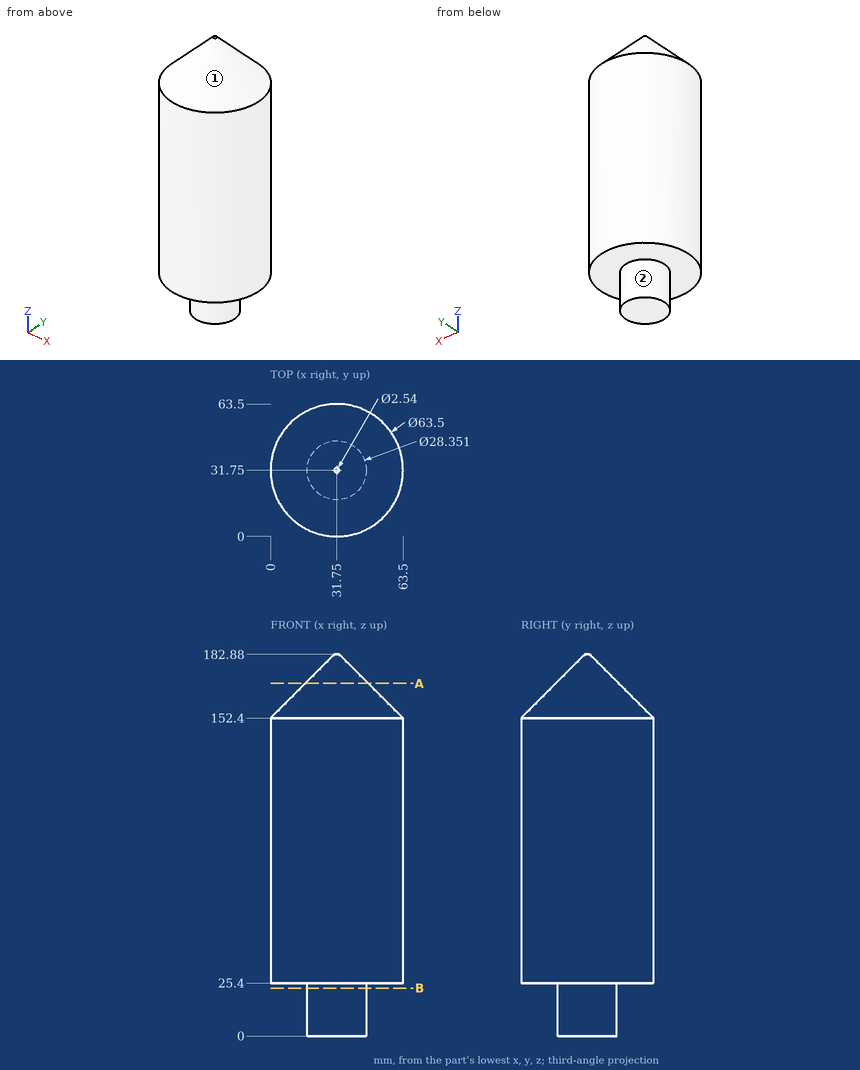
Study the drawing (mm; zero at the part's minimum x, y, z) and answer. A direction names the side the tool comes from. Round coordinates to 2 decimals unless told otherwise and drop trailing zeros. Write each loop counter-clockwise with the first axis right and the second up, starting at its lowest first coordinate (ties: lowest second). Pieces come first, ordered by that corner, then holes.
Q1. Straight lines are drawn through the part: line 1 (X direction, y = 27.5, z = 53); line 2 (X direction, y = 15.5, z = 92); line 3 (Z direction, x = 40, y = 46.5). For each, find the intervals that lie inside material, in ascending order.
Values:
line 1: x = 0.29 to 63.21
line 2: x = 4.47 to 59.03
line 3: z = 25.4 to 167.25
Q2. A tool of negligible diameter and unlimited length cuts with its end or side. For the marked faces 1 and 2, from which of +Z, -Z, +X, -X, +Y, -Y can it reach the whole face along a straight path? Write none if from no direction.
Values:
face 1: +Z
face 2: -Z
Q3. Find section A-A on z = 169. Determine the outline of the cut face in (x, y).
Values:
outline: circle Ø30.3 at (31.75, 31.75)
Q4. Flat-ended cylindrical pins translate along their axes: P1, Ø1.5, axis at x = 51.5, y = 44.5, coming from the -Z side; P2, Ø5, axis at x = 43.5, y = 12.5, coming from the +Z side; P3, Ø4, axis at x = 25, z = 18.5, coming from the +Y side. Find the tip coordinate at first contact, or state that the pin passes through.
Values:
P1: stops at z = 25.4
P2: stops at z = 164.1
P3: stops at y = 45.11
Q5. Find section B-B on z = 23. Determine the outline of the cut face in (x, y), and give its area (3 significant figures).
Values:
outline: circle Ø28.35 at (31.75, 31.75)
area: 631 mm2
